The listing builds one solid part. Answer for the finished solid, in the listing's coordinates (mm). A direction names the side the tool comes from. Coordinates: 2 decimals unless noted, no trailing zeros. Order: outer loops, then holes, each group sorted by start corner. A loop starts at its lowest first (then second) coordinate and runs counter-clockwise, first axis right, second up. Notation, with made-up numbers: M -26,-1.75 L 14,-1.75 A9 ccw 14,12.25 Z; hole C 77.5,2 d2. An arc over 180 degrees is marked long. One line per item, written item: value. Start each with the question number.
Q1. Straight lines are drawn through the part: line 1 along Y through (x, z) = (2.5, -100); line 2 along X through (y, z) = (2.5, -190); line 3 along Y through (x, z) = (51.5, -202.5). For each, find the intervals that lie inside material, in ascending order. Write a range as [from, to].
Q2. The part is cut by section A-A on x = 0. Give the vertices of the cut face in (y, z).
Q3. Determine the mould class of faces 5 (the cylindrical face through (-22.025, -99.184, -45.93)), 6 (the flat face through (0, -90, -41)), 7 (the flat face through (1, 15, -95)) for opening direction Y: pulls with the +Y half, pulls with the -Y half, needs draft (parallel to the pull), parting line crosses it, or undercut.
Q4. The part is cut by section B-B on z = -100. Give the vertices of the cut face in (x, y).
Q5. The part is cut by section D-D on x = 58. Give the vertices of the cut face in (y, z).
Q6. The part is cut by section C-C on y = 0. Give the vertices of the cut face in (x, z), then the cut area to 3 significant figures.
Q7. For faces 1 (the cylindrical face through (82.12, -34.05, -20.21)), 2 (the flat face through (-57, 0, -33)), 3 (the flat face through (0, 90, -51)), 4 (the flat face through (-1, -30, -123)), determine the directions among +Z, -Z, +X, -X, +Y, -Y from which every point of the face is accessible in a straight line to the end or side of a thin tool.
Q8. Each of these flat-tipped pins is pushed along its axis until it touches: pin 1 Ø15 at (y, z) = (3.5, -127) entering from -X; pin 2 Ø24 at (y, z) = (1, -94.5) entering from +X; pin 3 Ø6 at (y, z) = (55.5, -225) entering from -X. Where does it stop, or does it pass through?
```python
from build123d import *

# Parameters (mm, degrees)
SKETCH1_R           = 101.6
BOSS_EXTRUDE1_DEPTH = 250
CUT_EXTRUDE1_DEPTH  = 33
SKETCH4_R           = 101.6
SKETCH4_R_2         = 88.9
CUT_EXTRUDE2_DEPTH  = 41
CUT_EXTRUDE3_START  = -199
SKETCH5_R           = 101.6
SKETCH5_R_2         = 88.9
CUT_EXTRUDE3_DEPTH  = 199
SKETCH6_W           = 50
SKETCH6_H           = 30
CUT_EXTRUDE4_DEPTH  = 287


with BuildPart() as part:
    # Sketch1 → Boss-Extrude1 (new body)
    with BuildSketch(Plane.XY):
        Circle(SKETCH1_R)
    extrude(amount=-BOSS_EXTRUDE1_DEPTH)

    # Sketch2 → Cut-Extrude1 (cut)
    with BuildSketch(Plane.XY):
        with BuildLine():
            Line((87.625395862, 15), (-87.625395862, 15))
            ThreePointArc((-87.625395862, 15), (-88.9, 0), (-87.625395862, -15))
            Line((-87.625395862, -15), (87.625395862, -15))
            ThreePointArc((87.625395862, -15), (88.580775827, -7.527028227), (88.9, 0))
            ThreePointArc((88.9, 0), (88.580775827, 7.527028227), (87.625395862, 15))
        make_face()
    extrude(amount=-CUT_EXTRUDE1_DEPTH, mode=Mode.SUBTRACT)

    # Sketch4 → Cut-Extrude2 (cut)
    with BuildSketch(Plane.XY):
        Circle(SKETCH4_R)
        Circle(SKETCH4_R_2, mode=Mode.SUBTRACT)
    extrude(amount=-CUT_EXTRUDE2_DEPTH, mode=Mode.SUBTRACT)

    # Sketch5 → Cut-Extrude3 (cut)
    with BuildSketch(Plane(origin=(0, 0, -250), x_dir=(-1, 0, 0), z_dir=(0, 0, -1)).offset(CUT_EXTRUDE3_START)):
        with Locations(Location((0, 0, 0), (0, 0, 180))):
            Circle(SKETCH5_R)
        with Locations(Location((0, 0, 0), (0, 0, 180))):
            Circle(SKETCH5_R_2, mode=Mode.SUBTRACT)
    extrude(amount=CUT_EXTRUDE3_DEPTH, mode=Mode.SUBTRACT)

    # Sketch6 → Cut-Extrude4 (cut)
    with BuildSketch(Plane.XY):
        with BuildLine():
            Line((-71.45802964, 30), (71.45802964, 30))
            ThreePointArc((71.45802964, 30), (0, 77.5), (-71.45802964, 30))
        make_face()
        with BuildLine():
            Line((-71.45802964, -30), (71.45802964, -30))
            ThreePointArc((71.45802964, -30), (0, -77.5), (-71.45802964, -30))
        make_face()
        Rectangle(SKETCH6_W, SKETCH6_H)
    extrude(amount=-CUT_EXTRUDE4_DEPTH, mode=Mode.SUBTRACT)


solid = part.part
```
Output:
1. line 1: y = [-88.86, -77.46], [-30, -15], [15, 30], [77.46, 88.86]
1. line 2: x = [-88.86, -25], [25, 88.86]
1. line 3: y = [-72.46, -57.91], [-30, 30], [57.91, 72.46]
2. outline: M -101.6,-51 L -88.9,-51 L -88.9,-250 L -77.5,-250 L -77.5,0 L -88.9,0 L -88.9,-41 L -101.6,-41 Z; M -30,-250 L -15,-250 L -15,0 L -30,0 Z; M 15,-250 L 30,-250 L 30,0 L 15,0 Z; M 77.5,-250 L 88.9,-250 L 88.9,-51 L 101.6,-51 L 101.6,-41 L 88.9,-41 L 88.9,0 L 77.5,0 Z
3. face 5: parting line crosses it
3. face 6: needs draft
3. face 7: undercut
4. outline: C 0,0 d177.8; hole M -71.46,-30 A77.5 ccw 71.46,-30 Z; hole M -71.46,30 L 71.46,30 A77.5 ccw Z; hole M -25,-15 L 25,-15 L 25,15 L -25,15 Z
5. outline: M -83.42,-51 L -67.37,-51 L -67.37,-250 L -51.4,-250 L -51.4,0 L -67.37,0 L -67.37,-41 L -83.42,-41 Z; M -30,-250 L 30,-250 L 30,0 L 15,0 L 15,-33 L -15,-33 L -15,0 L -30,0 Z; M 51.4,-250 L 67.37,-250 L 67.37,-51 L 83.42,-51 L 83.42,-41 L 67.37,-41 L 67.37,0 L 51.4,0 Z
6. outline: M -101.6,-51 L -88.9,-51 L -88.9,-250 L -25,-250 L -25,-33 L -88.9,-33 L -88.9,-41 L -101.6,-41 Z; M 25,-250 L 88.9,-250 L 88.9,-51 L 101.6,-51 L 101.6,-41 L 88.9,-41 L 88.9,-33 L 25,-33 Z
6. area: 28,000 mm^2
7. face 1: +Z
7. face 2: +Z, +X, -X
7. face 3: -Z
7. face 4: +Z, -Z
8. pin 1: stops at x = -88.9
8. pin 2: stops at x = 88.9
8. pin 3: stops at x = -71.74
